```python
from build123d import *

# Parameters (mm, degrees)
SKETCH1_W               = 1216.025
SKETCH1_H               = 1190.625
BOSS_EXTRUDE1_DEPTH     = 17.8562
SKETCH3_R               = 55
CUT_EXTRUDE1_DEPTH      = 1
CUT_EXTRUDE1_DEPTH_BACK = 18.8562
SKETCH4_R               = 4.25
CUT_EXTRUDE2_DEPTH      = 1
CUT_EXTRUDE2_DEPTH_BACK = 18.8562
SKETCH5_R               = 1.3890625
CUT_EXTRUDE3_DEPTH      = 1
CUT_EXTRUDE3_DEPTH_BACK = 18.8562
SKETCH10_R              = 3.571875
CUT_EXTRUDE4_DEPTH      = 1
CUT_EXTRUDE4_DEPTH_BACK = 18.8562


with BuildPart() as part:
    # Sketch1 → Boss-Extrude1 (new body)
    with BuildSketch(Plane(origin=(0, 0, 0), x_dir=(1, 0, 0), z_dir=(0, 1, 0))):
        with Locations((608.0125, -595.3125)):
            Rectangle(SKETCH1_W, SKETCH1_H)
    extrude(amount=BOSS_EXTRUDE1_DEPTH)

    # Sketch3 → Cut-Extrude1 (cut, two sides)
    with BuildSketch(Plane(origin=(0, 17.8562, 0), x_dir=(1, 0, 0), z_dir=(0, 1, 0))) as cut_extrude1_sk:
        with Locations((608.0125, -595.376)):
            Circle(SKETCH3_R)
    extrude(amount=CUT_EXTRUDE1_DEPTH, mode=Mode.SUBTRACT)
    extrude(cut_extrude1_sk.sketch, amount=-CUT_EXTRUDE1_DEPTH_BACK, mode=Mode.SUBTRACT)

    # Sketch4 → Cut-Extrude2 (cut, two sides)
    with BuildSketch(Plane(origin=(0, 17.8562, 0), x_dir=(1, 0, 0), z_dir=(0, 1, 0))) as cut_extrude2_sk:
        with Locations((562.050559223, -549.414059223)):
            Circle(SKETCH4_R)
        with Locations((653.974440777, -549.414059223)):
            Circle(SKETCH4_R)
        with Locations((653.974440777, -641.337940777)):
            Circle(SKETCH4_R)
        with Locations((562.050559223, -641.337940777)):
            Circle(SKETCH4_R)
    extrude(amount=CUT_EXTRUDE2_DEPTH, mode=Mode.SUBTRACT)
    extrude(cut_extrude2_sk.sketch, amount=-CUT_EXTRUDE2_DEPTH_BACK, mode=Mode.SUBTRACT)

    # Sketch5 → Cut-Extrude3 (cut, two sides)
    with BuildSketch(Plane(origin=(0, 17.8562, 0), x_dir=(1, 0, 0), z_dir=(0, 1, 0))) as cut_extrude3_sk:
        with Locations((12.7, -12.7)):
            Circle(SKETCH5_R)
        with Locations((12.7, -63.5)):
            Circle(SKETCH5_R)
        with Locations((63.5, -12.7)):
            Circle(SKETCH5_R)
        with Locations((12.7, -114.3)):
            Circle(SKETCH5_R)
        with Locations((114.3, -12.7)):
            Circle(SKETCH5_R)
        with Locations((12.7, -241.3)):
            Circle(SKETCH5_R)
        with Locations((12.7, -368.3)):
            Circle(SKETCH5_R)
        with Locations((12.7, -495.3)):
            Circle(SKETCH5_R)
        with Locations((241.3, -12.7)):
            Circle(SKETCH5_R)
        with Locations((368.3, -12.7)):
            Circle(SKETCH5_R)
        with Locations((495.3, -12.7)):
            Circle(SKETCH5_R)
        with Locations((720.725, -12.7)):
            Circle(SKETCH5_R)
        with Locations((847.725, -12.7)):
            Circle(SKETCH5_R)
        with Locations((974.725, -12.7)):
            Circle(SKETCH5_R)
        with Locations((1203.325, -495.3)):
            Circle(SKETCH5_R)
        with Locations((1203.325, -368.3)):
            Circle(SKETCH5_R)
        with Locations((1203.325, -241.3)):
            Circle(SKETCH5_R)
        with Locations((1101.725, -12.7)):
            Circle(SKETCH5_R)
        with Locations((1203.325, -114.3)):
            Circle(SKETCH5_R)
        with Locations((1152.525, -12.7)):
            Circle(SKETCH5_R)
        with Locations((1203.325, -63.5)):
            Circle(SKETCH5_R)
        with Locations((1203.325, -12.7)):
            Circle(SKETCH5_R)
        with Locations((1203.325, -1177.925)):
            Circle(SKETCH5_R)
        with Locations((1203.325, -1127.125)):
            Circle(SKETCH5_R)
        with Locations((1152.525, -1177.925)):
            Circle(SKETCH5_R)
        with Locations((1203.325, -1076.325)):
            Circle(SKETCH5_R)
        with Locations((1101.725, -1177.925)):
            Circle(SKETCH5_R)
        with Locations((1203.325, -949.325)):
            Circle(SKETCH5_R)
        with Locations((1203.325, -822.325)):
            Circle(SKETCH5_R)
        with Locations((1203.325, -695.325)):
            Circle(SKETCH5_R)
        with Locations((974.725, -1177.925)):
            Circle(SKETCH5_R)
        with Locations((847.725, -1177.925)):
            Circle(SKETCH5_R)
        with Locations((720.725, -1177.925)):
            Circle(SKETCH5_R)
        with Locations((495.3, -1177.925)):
            Circle(SKETCH5_R)
        with Locations((368.3, -1177.925)):
            Circle(SKETCH5_R)
        with Locations((241.3, -1177.925)):
            Circle(SKETCH5_R)
        with Locations((12.7, -695.325)):
            Circle(SKETCH5_R)
        with Locations((12.7, -822.325)):
            Circle(SKETCH5_R)
        with Locations((12.7, -949.325)):
            Circle(SKETCH5_R)
        with Locations((114.3, -1177.925)):
            Circle(SKETCH5_R)
        with Locations((12.7, -1076.325)):
            Circle(SKETCH5_R)
        with Locations((63.5, -1177.925)):
            Circle(SKETCH5_R)
        with Locations((12.7, -1127.125)):
            Circle(SKETCH5_R)
        with Locations((12.7, -1177.925)):
            Circle(SKETCH5_R)
    extrude(amount=CUT_EXTRUDE3_DEPTH, mode=Mode.SUBTRACT)
    extrude(cut_extrude3_sk.sketch, amount=-CUT_EXTRUDE3_DEPTH_BACK, mode=Mode.SUBTRACT)

    # Sketch10 → Cut-Extrude4 (cut, two sides)
    with BuildSketch(Plane(origin=(0, 17.8562, 0), x_dir=(1, 0, 0), z_dir=(0, 1, 0))) as cut_extrude4_sk:
        with Locations((173.0375, -682.625)):
            Circle(SKETCH10_R)
        with Locations((233.3625, -682.625)):
            Circle(SKETCH10_R)
        with Locations((350.8375, -152.4)):
            Circle(SKETCH10_R)
        with Locations((411.1625, -152.4)):
            Circle(SKETCH10_R)
        with Locations((804.8625, -152.4)):
            Circle(SKETCH10_R)
        with Locations((865.1875, -152.4)):
            Circle(SKETCH10_R)
        with Locations((982.6625, -682.625)):
            Circle(SKETCH10_R)
        with Locations((1042.9875, -682.625)):
            Circle(SKETCH10_R)
    extrude(amount=CUT_EXTRUDE4_DEPTH, mode=Mode.SUBTRACT)
    extrude(cut_extrude4_sk.sketch, amount=-CUT_EXTRUDE4_DEPTH_BACK, mode=Mode.SUBTRACT)


solid = part.part
```
Here's how the part is built. I have some questions about the finished solid (model axes, mm). Coordinates: 2 decimals unless noted, no trailing zeros. Order: outer loops, then holes, each group sorted by start corner. A loop starts at its lowest first (then second) coordinate and runs counter-clockwise, first axis right, second up. Notation, with made-up numbers: M 14.5,52.25 L 58.5,52.25 A6 cw 58.5,56.25 Z; hole C 81.25,38.25 d8. An arc over 180 degrees is marked long. Answer as a JSON object with one key per item and string values. Group by question number.
(1) For pin 1 (1.7 mm diameter, centred on x = 1203.325, z = 114.3, fed in from +Y), with a flat end and sliding along its axis, tell me the tip position at first contact or that it passes through.
(2) Suppose I cut it at A-A, the plane z = 574. Please give me the cut outline in (x, y) (3 decimals), then the cut area to 3 significant figures.
(3) If we mould it in two halves opening along Z, with no side actions, what happens to faces 1 (the face through (564.366, 9.053, 628.843)), 2 (the face through (600, 17.856, 455))? For each: released by +Z, released by -Z, zero draft, split by the parting line, or undercut.
(4) I need wall thicknesses on probe 1 along X at (y, z) = (14.75, 695.5) (3 decimals); probe 2 along Z at (x, y) = (561.5, 5.25) (3 decimals); probe 3 along Z at (x, y) = (1041.5, 15.75) (3 decimals). Which ranges of each line are inside material? Lowest first, please.
Values found:
{
 "1": {"pin 1": "passes through"},
 "2": {"outline": "M 0,0 L 557.336,0 L 557.336,17.856 L 0,17.856 Z; M 658.689,0 L 1216.025,0 L 1216.025,17.856 L 658.689,17.856 Z", "area": "19,900 mm^2"},
 "3": {"face 1": "undercut", "face 2": "zero draft"},
 "4": {"probe 1": "x = 0 to 11.322, 14.078 to 1201.947, 1204.703 to 1216.025", "probe 2": "z = 0 to 545.2, 553.628 to 566.023, 624.729 to 637.124, 645.552 to 1190.625", "probe 3": "z = 0 to 679.378, 685.872 to 1190.625"}
}
